Source: CAD feature listing. Evaluate the final solid. Frame: model axes, mm. A direction names the side the tool comes from. Coordinates: 2 decimals unless noted, no trailing zeros. Loops run counter-clockwise (first coordinate to the right, second up) from the corner with the lowest first, then second, coordinate; pieces in that order, holes last. Notation, with made-up numbers: (-3, -7.5) -> (27, -7.5) arc R13 ccw to (27, -2.5) -> close; hole circle Ø4 at (11, 60.5). An arc over 180 degrees is marked (long way). One line per question, with ' | ' between items. Start each with the question number.
Autodesk Inventor part; units mm, degrees
ref_plane "YZ Plane" through (0, 0, 0) normal (1, 0, 0) x (0, 1, 0)
ref_plane "XZ Plane" through (0, 0, 0) normal (0, 1, 0) x (-1, 0, 0)
ref_plane "XY Plane" through (0, 0, 0) normal (0, 0, 1) x (1, 0, 0)
sketch "Sketch1" plane through (0, 0, 0) normal (1, 0, 0) x (0, 1, 0)
  line L0 (0, 4.5482) -> (0, -51.0669)
  line L1 (0, -51.0669) -> (8.138, -51.0669)
  line L2 (8.138, -51.0669) -> (8.138, -37.701)
  line L3 (8.138, -37.701) -> (37.1169, -37.701)
  line L4 (37.1169, -37.701) -> (37.1169, -8.8176)
  line L5 (37.1169, -8.8176) -> (8.138, -8.8176)
  line L6 (8.138, -8.8176) -> (8.138, 4.5482)
  line L7 (8.138, 4.5482) -> (0, 4.5482)
  line L8 (37.1169, -23.2593) -> (0, -23.2593) construction
  circle A0 centre (22.1376, -23.2593) radius 10.9855
  dimension "d0" = 21.971
extrude "Extrusion1" add sketch "Sketch1" along normal blind 19.05
fillet "Fillet1" radius 3.175 6 edges at (9.525, 37.1169, -8.8176) (9.525, 8.138, -8.8176) (9.525, 37.1169, -37.701) (9.525, 8.138, -37.701) (9.525, 8.138, -51.0669) (9.525, 8.138, 4.5482)
sketch "Sketch2" plane through (0, 8.138, -40.876) normal (0, 1, 0) x (1, 0, 0)
  line L0 (0, 7.0159) -> (19.05, 7.0159)
  line L1 (0, 7.0159) -> (0, 0)
  line L2 (19.05, 0) -> (0, 0)
  line L3 (19.05, 7.0159) -> (19.05, 0)
  line L4 (19.05, -42.2493) -> (0, -42.2493)
  line L5 (19.05, -35.2334) -> (19.05, -42.2493)
  line L6 (0, -35.2334) -> (19.05, -35.2334)
  line L7 (0, -35.2334) -> (0, -42.2493)
  line L8 (0, 7.0159) -> (19.05, 7.0159) construction
  line L9 (9.525, 7.0159) -> (9.525, 0) construction
  line L10 (0, -35.2334) -> (19.05, -35.2334) construction
  line L11 (9.525, -35.2334) -> (9.525, -42.2493) construction
  circle A0 centre (9.525, 3.5079) radius 1.5356
  circle A1 centre (9.525, -38.7413) radius 1.5356
  point P0 (0, -40.876)
  dimension "d4" = 3.0712
extrude "Extrusion2" cut sketch "Sketch2" against normal through all contours A0 | A1
fillet "Fillet2" radius 1.5875 1 edges at (0, 11.1521, -23.2593)
properties part number "bearing holder"
(1) Draft query along X for faces 4 (the cylindrical face through (9.658, 7.233, 3.593)), 5 (the cylindrical face through (9.325, 4.126, -45.906)), 6 (the flat face through (0, 10, -17)). Return one class per face: pulls with the +X half, pulls with the -X half, needs draft (parallel to the pull), parting line crosses it, or undercut.
(2) Access query for faces 1 (the flat face through (9, 8.138, -46)), 2 (the flat face through (9, 8.138, -4)), 3 (the flat face through (19.05, 10, -23)). Directions: +Z, -Z, +X, -X, +Y, -Y. A direction counts if a zero-diameter tool reaches every point of the face in a straight line with its end or side. Return the directions, or none.
(3) Cut plane B-B, the plane z = -45. Return the cut outline in (x, y), and give its area (3 significant figures).
(4) Contact query for flat-ended pins moving along their axis: pin 1 Ø3 at (x, y) = (13, 11.5) entering from -Z; pin 2 Ø5.5 at (x, z) = (7, -1) entering from +Y; pin 3 Ø5 at (x, y) = (10, 29.5) entering from -Z. Output: stop coordinate, or through.
(5) Cut plane A-A, the plane x = 10.5. State how many separate pieces and enclosed holes the cut face has, and give its area (3 significant figures).
(6) Ray query, L1, parallel to Y at x = 8.25, z = -27.5; L2, parallel to Z at x = 2.25, y = 16; L3, parallel to Z at x = 7.75, y = 23. Return the intervals inside material, ascending.
(7) Cut plane D-D, the plane y = 35.5. Return the cut outline in (x, z).
Here are the results:
1) face 4: needs draft | face 5: undercut | face 6: pulls with the -X half
2) face 1: -Z, +X, -X, +Y | face 2: +Z, +X, -X, +Y | face 3: +Z, -Z, +X, +Y, -Y
3) outline: (0, 0) -> (8.12, 0) -> (8.12, 8.14) -> (0, 8.14) -> close; (10.93, 0) -> (19.05, 0) -> (19.05, 8.14) -> (10.93, 8.14) -> close | area: 132 mm2
4) pin 1: stops at z = -37.99 | pin 2: stops at y = 8.14 | pin 3: stops at z = -37.7
5) separate pieces: 3 | enclosed holes: 1 | area: 868 mm2
6) L1: y = 0 to 12, 32.27 to 37.12 | L2: z = -37.7 to -32.37, -14.15 to -8.82 | L3: z = -37.7 to -34.21, -12.31 to -8.82
7) outline: (0, -37.29) -> (19.05, -37.29) -> (19.05, -9.23) -> (0, -9.23) -> close
